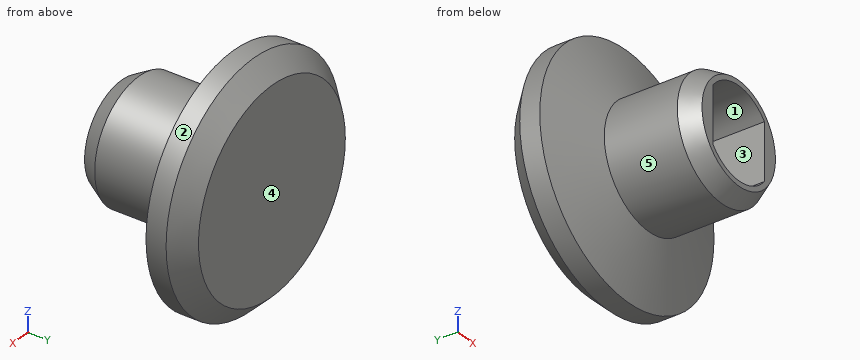
from build123d import *

# Parameters (mm, degrees)
CUT_EXTRUDE1_DEPTH = 5.5
CHAMFER1_SIZE      = 0.5
CHAMFER1_SIZE2     = 0.866025404


with BuildPart() as part:
    # Sketch1 → Revolve1 (revolve)
    with BuildSketch(Plane.XY):
        Polygon((0, 0), (0, 7.5), (-5, 7.5), (-5.932615316, 6.567384684), (-5.932615316, 5.567384684), (-3, 4.5), (-3, 0), align=None)
    revolve(axis=Axis((0, 14, 0), (0, -1, 0)))

    # Sketch2 → Cut-Extrude1 (cut)
    with BuildSketch(Plane.XZ):
        with BuildLine():
            Line((1.75, -1.414213562), (1.75, 1.414213562))
            ThreePointArc((1.75, 1.414213562), (0, 2.25), (-1.75, 1.414213562))
            Line((-1.75, 1.414213562), (-1.75, -1.414213562))
            ThreePointArc((-1.75, -1.414213562), (0, -2.25), (1.75, -1.414213562))
        make_face()
    extrude(amount=-CUT_EXTRUDE1_DEPTH, mode=Mode.SUBTRACT)

    # Chamfer1
    chamfer1_edges = [part.edges().sort_by_distance(p)[0] for p in [
        (3, 0, 0),
    ]]
    chamfer1_side = [part.faces().sort_by_distance(p)[0] for p in [
        (2.915147186, 0, 0),
    ]]
    chamfer(chamfer1_edges, length=CHAMFER1_SIZE, length2=CHAMFER1_SIZE2, reference=chamfer1_side[0])


solid = part.part
The listing builds one solid part. Answer for the finished solid, in the listing's coordinates (mm). Face numbers are marked on the shaded views. A direction names the side the tool comes from. Round coordinates to 2 decimals unless told otherwise and drop trailing zeros. Write each loop counter-clockwise with the first axis right and the second up, starting at its lowest first coordinate (ties: lowest second). Pieces come first, ordered by that corner, then holes. Notation, with made-up numbers: (18, -12.5) - (58, -12.5) arc R17 ccw to (58, 11.5) - close; hole circle Ø7 at (40, 34). An arc over 180 degrees is marked (long way). Use one line per item in the form item = value. Start each with the question number.
Item 1: Flat-ended cylindrical pins translate along their axes: pin 1 Ø3 at (y, z) = (5, -4.5) entering from -X; pin 2 Ø2 at (x, z) = (3.5, -4.5) entering from +Y; pin 3 Ø2 at (y, z) = (2.5, 3.5) entering from -X; pin 4 Ø2.5 at (y, z) = (2, 0.5) entering from +X. Find the tip coordinate at first contact, or state that the pin passes through.
Item 2: A cutting plane is placed at A-A (z = 0). Write down the section's boundary in (x, y), plus the area to 3 significant figures.
Item 3: Find the intervals of material crossed by line 1 (X direction, y = 1.5, z = -1.5); line 2 (X direction, y = 2.5, z = -1); line 3 (Y direction, x = 1.25, z = -0.75), in increasing order. Write a range as [from, to].
Item 4: A tool of negligible diameter and unlimited length cuts with its end or side. For the marked faces 1 and 2, from which of +Z, -Z, +X, -X, +Y, -Y can it reach the whole face along a straight path? Write none if from no direction.
Item 5: A cutting plane is placed at D-D (y = 6.25). Write down the section's boundary in (x, z).
Item 6: A cutting plane is placed at B-B (x = 0). Write down the section's boundary in (y, z), plus the area to 3 significant figures.
Item 7: A cutting plane is placed at C-C (y = 1.75). Write down the section's boundary in (x, z).
Item 8: Determine the mould class of the marked faces 3, 4 and 5 for opening direction X: +X half, -X half, draft (parallel to the pull), parting line (faces both ways), or undercut.
The answers:
q1.pin_1 = -5.05
q1.pin_2 = 7.5
q1.pin_3 = -1.66
q1.pin_4 = 3
q2.outline = (-5.93, 5.57) - (-3, 4.5) - (-3, 0.87) - (-2.5, 0) - (-1.75, 0) - (-1.75, 5.5) - (1.75, 5.5) - (1.75, 0) - (2.5, 0) - (3, 0.87) - (3, 4.5) - (5.93, 5.57) - (5.93, 6.57) - (5, 7.5) - (-5, 7.5) - (-5.93, 6.57) - close
q2.area = 38.9 mm^2
q3.line_1 = [-2.6, -1.68], [1.68, 2.6]
q3.line_2 = [-2.83, -1.75], [1.75, 2.83]
q3.line_3 = [5.5, 7.5]
q4.face_1 = -Y
q4.face_2 = +Y, -Y
q5.outline = circle Ø11.87 at (0, 0)
q6.outline = (0, -2.5) - (0.87, -3) - (4.5, -3) - (5.57, -5.93) - (6.57, -5.93) - (7.5, -5) - (7.5, 5) - (6.57, 5.93) - (5.57, 5.93) - (4.5, 3) - (0.87, 3) - (0, 2.5) - (0, 2.25) - (5.5, 2.25) - (5.5, -2.25) - (0, -2.25) - close
q6.area = 33.4 mm^2
q7.outline = circle Ø6 at (0, 0); hole (-1.75, -1.41) arc R2.25 ccw to (1.75, -1.41) - (1.75, 1.41) arc R2.25 ccw to (-1.75, 1.41) - close
q8.face_3 = undercut
q8.face_4 = draft
q8.face_5 = parting line
